Build history of the part. All positions in model axes, mm. Give positions to 0.01 mm unless a question says otherwise; leave off trailing zeros. Order: outer loops, then holes, each group sorted by start corner. A loop starts at its lowest first (then second) coordinate and runs counter-clockwise, first axis right, second up. Notation, with made-up numbers: M 10,-1 L 50,-1 A21 ccw 50,10 Z; hole C -1.75,-25 d3. An arc over 180 degrees is marked long. One line per item, written item: value. Start each with the question number.
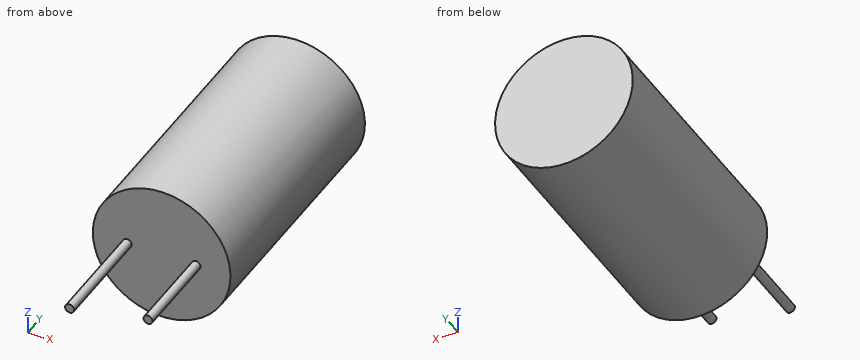
from build123d import *

# Parameters (mm, degrees)
SKETCH_1_R      = 7.62
EXTRUDE_1_DEPTH = 28
SKETCH_2_R      = 0.5
EXTRUDE_2_DEPTH = 12
SKETCH_3_R      = 0.5
EXTRUDE_3_DEPTH = 10


with BuildPart() as part:
    # 草图1 → 拉伸1 (new body)
    with BuildSketch(Plane(origin=(0, 0, 0), x_dir=(1, 0, 0), z_dir=(0, 1, 0))):
        with Locations(Location((0, 0, 0), (0, 0, 270))):
            Circle(SKETCH_1_R)
    extrude(amount=EXTRUDE_1_DEPTH)

    # 草图2 → 拉伸2 (add)
    with BuildSketch(Plane.XZ):
        with Locations(Location((-3.81, 0, 0), (0, 0, 90))):
            Circle(SKETCH_2_R)
    extrude(amount=EXTRUDE_2_DEPTH)

    # 草图3 → 拉伸3 (add)
    with BuildSketch(Plane.XZ):
        with Locations(Location((3.81, 0, 0), (0, 0, 90))):
            Circle(SKETCH_3_R)
    extrude(amount=EXTRUDE_3_DEPTH)


solid = part.part
1) Slice it at A-A (z = 0). List the corners of the cut face in (x, y), plus the area to 3 significant figures.
2) Drill centre lines: line 1 (Y direction, x = 6, z = 3.25); line 2 (Z direction, x = -2.5, y = 24.5); line 3 (Z direction, x = 6.5, y = 25). Where is each one in solid material? Low to high.
3) Slice it at D-D (y = 2). List the corners of the cut face in (x, z).
4) Drop flat-ended pins along their axis: P1, Ø4.5, axis at x = 0.5, z = 3.5, coming from the -Y side; P2, Ø8, axis at x = 6, y = 22.5, coming from the +Z side; P3, Ø1.5, axis at y = 12.5, z = -4.5, coming from the -X side. Give the stop position or say it passes through.
5) Slice it at C-C (y = -7.5). List the corners of the cut face in (x, z).
6) Slice it at B-B (x = -3.81). List the corners of the cut face in (y, z).
Results list:
1. outline: M -7.62,0 L -4.31,0 L -4.31,-12 L -3.31,-12 L -3.31,0 L 3.31,0 L 3.31,-10 L 4.31,-10 L 4.31,0 L 7.62,0 L 7.62,28 L -7.62,28 Z
1. area: 449 mm²
2. line 1: y = 0 to 28
2. line 2: z = -7.2 to 7.2
2. line 3: z = -3.98 to 3.98
3. outline: C 0,0 d15.24
4. P1: stops at y = 0
4. P2: stops at z = 7.35
4. P3: stops at x = -6.63
5. outline: C -3.81,0 d1; C 3.81,0 d1
6. outline: M -12,-0.5 L 0,-0.5 L 0,-6.6 L 28,-6.6 L 28,6.6 L 0,6.6 L 0,0.5 L -12,0.5 Z
